Autodesk Inventor part; units mm, degrees
ref_plane "YZ Plane" through (0, 0, 0) normal (1, 0, 0) x (0, 1, 0)
ref_plane "XZ Plane" through (0, 0, 0) normal (0, 1, 0) x (-1, 0, 0)
ref_plane "XY Plane" through (0, 0, 0) normal (0, 0, 1) x (1, 0, 0)
sketch "Sketch1" plane through (0, 0, 0) normal (0, 0, 1) x (1, 0, 0)
  line L0 (-50, 10) -> (50, 10) construction
  line L1 (50, 10) -> (50, -10) construction
  line L2 (50, -10) -> (-50, -10) construction
  line L3 (-50, -10) -> (-50, 10) construction
  line L4 (-50, 10) -> (50, -10) construction
  line L5 (50, 10) -> (-50, -10) construction
  line L6 (10, -30) -> (-10, -30) construction
  line L7 (-10, -30) -> (-10, 30) construction
  line L8 (-10, 30) -> (10, 30) construction
  line L9 (10, 30) -> (10, -30) construction
  line L10 (10, -30) -> (-10, 30) construction
  line L11 (-10, -30) -> (10, 30) construction
  line L12 (-50, 10) -> (-10, 30)
  line L13 (-10, 30) -> (10, 30)
  line L14 (10, 30) -> (50, 10)
  line L15 (50, 10) -> (50, -10)
  line L16 (50, -10) -> (10, -30)
  line L17 (10, -30) -> (-10, -30)
  line L18 (-10, -30) -> (-50, -10)
  line L19 (-50, -10) -> (-50, 10)
  point P0 (0, 0)
  dimension "d0" = 20
  dimension "d2" = 100
  dimension "d3" = 20
  dimension "d4" = 60
extrude "Extrusion1" add sketch "Sketch1" along normal mid plane 4
sketch "Sketch2" plane through (0, 0, 2) normal (0, 0, 1) x (1, 0, 0)
  line L0 (-50, 10) -> (-50, -10)
  line L1 (-10, -30) -> (10, -30)
  line L2 (50, -10) -> (50, 10)
  line L3 (10, 30) -> (-10, 30)
  line L4 (0, 30) -> (0, -30) construction
  line L5 (-50, 0) -> (50, 0) construction
  point P0 (0, 0)
  point P1 (0, 0)
  point P2 (20, 0)
  point P3 (40, 0)
  point P4 (0, 20)
  point P5 (0, -20)
  point P6 (-20, 0)
  point P7 (-40, 0)
  dimension "d7" = 20
  dimension "d9" = 20
  dimension "d10" = 20
  dimension "d11" = 20
  dimension "d12" = 20
  dimension "d13" = 20
hole "Hole1" at (0, 0, 2) at (20, 0, 2) at (40, 0, 2) at (0, 20, 2) at (0, -20, 2) at (-20, 0, 2) at (-40, 0, 2) direction (0, 0, -1) diameter 5 end through all
properties part number "7 Hole Cross Joining Plate" material "Aluminum 6061"
Source: CAD feature listing. Evaluate the final solid. Frame: model axes, mm. Give positions to 0.01 mm unless a question says otherwise; leave off trailing zeros. Write each loop counter-clockwise with the first axis right and the second up, starting at its lowest first coordinate (ties: lowest second). Pieces come first, ordered by that corner, then holes. Notation, with made-up numbers: M -33.5,-11 L -6.5,-11 A24 cw -6.5,24 Z; hole C 2,8.25 d3. An arc over 180 degrees is marked long. Return JSON: item names as keys, results as strings. Group by question number.
1) Draft query along Y for faces 1 (the face through (-0.1, 22.5, 0)), 2 (the face through (-30, 20, 0)), 3 (the face through (-30, -20, 0)), 4 (the face through (-1, -6, -2)). Return one class per face: released by +Y, released by -Y, zero draft, split by the parting line, or undercut.
2) Cut plane A-A, the plane y = -20. Output: boundary loops of the cut face in (x, z).
3) Cut plane D-D, the plane z = -1.1. Output: boundary loops of the cut face in (x, y).
4) Cut plane B-B, the plane x = 20. Output: boundary loops of the cut face in (y, z).
5) Ray query, L1, parallel to Y at x = 0, z = 0.35; L2, parallel to X at y = 0, z = 0.95; L3, parallel to X at y = 20, z = -0.2. Return the intervals inside material, ascending.
6) Cut plane C-C, the plane y = 0. Output: boundary loops of the cut face in (x, z), then the cut area to 3 significant figures.
7) First-contact query: pin 1 Ø1.5 at (y, z) = (-17, -1.5) entering from +X; pin 2 Ø2 at (y, z) = (-18.5, 0.5) entering from -X. Flat tips, straight axial feed; report the tip coordinate or a pass-through.
Data:
{
 "1": {"face 1": "undercut", "face 2": "released by +Y", "face 3": "released by -Y", "face 4": "zero draft"},
 "2": {"outline": "M -30,-2 L -2.5,-2 L -2.5,2 L -30,2 Z; M 2.5,-2 L 30,-2 L 30,2 L 2.5,2 Z"},
 "3": {"outline": "M -50,-10 L -10,-30 L 10,-30 L 50,-10 L 50,10 L 10,30 L -10,30 L -50,10 Z; hole C -40,0 d5; hole C -20,0 d5; hole C 0,-20 d5; hole C 0,0 d5; hole C 0,20 d5; hole C 20,0 d5; hole C 40,0 d5"},
 "4": {"outline": "M -25,-2 L -2.5,-2 L -2.5,2 L -25,2 Z; M 2.5,-2 L 25,-2 L 25,2 L 2.5,2 Z"},
 "5": {"L1": "y = -30 to -22.5, -17.5 to -2.5, 2.5 to 17.5, 22.5 to 30", "L2": "x = -50 to -42.5, -37.5 to -22.5, -17.5 to -2.5, 2.5 to 17.5, 22.5 to 37.5, 42.5 to 50", "L3": "x = -30 to -2.5, 2.5 to 30"},
 "6": {"outline": "M -50,-2 L -42.5,-2 L -42.5,2 L -50,2 Z; M -37.5,-2 L -22.5,-2 L -22.5,2 L -37.5,2 Z; M -17.5,-2 L -2.5,-2 L -2.5,2 L -17.5,2 Z; M 2.5,-2 L 17.5,-2 L 17.5,2 L 2.5,2 Z; M 22.5,-2 L 37.5,-2 L 37.5,2 L 22.5,2 Z; M 42.5,-2 L 50,-2 L 50,2 L 42.5,2 Z", "area": "300 mm²"},
 "7": {"pin 1": "stops at x = 37.5", "pin 2": "stops at x = -35"}
}
